Could you check a few things on this model? Use its own coordinates, in mm. A direction names the side the tool comes from. Give positions to 0.01 mm unless a question says otherwise; leave off trailing zeros. Order: outer loops, then holes, each group sorted by start corner. A loop starts at its lowest first (then second) coordinate and runs counter-clockwise, first axis right, second up. Notation, with made-up numbers: (-23.5, 31.5) -> (2.5, 31.5) arc R19 cw to (2.5, 36.5) -> close; hole circle Ø6 at (3, -26.75). An arc over 180 degrees is marked (long way). Write each question's results on one line, items separated by ' | '.
Autodesk Inventor part; units mm, degrees
ref_plane "YZ Plane" through (0, 0, 0) normal (1, 0, 0) x (0, 1, 0)
ref_plane "XZ Plane" through (0, 0, 0) normal (0, 1, 0) x (-1, 0, 0)
ref_plane "Work Plane1" through (0, 0, -3) normal (0, 0, 1) x (1, 0, 0)
sketch "Sketch1" plane through (0, 0, 0) normal (0, 0, 1) x (1, 0, 0)
  circle A0 centre (-6.35, 0) radius 3.885
  circle A1 centre (6.35, 0) radius 3.885
  arc A2 (-4.5733, 3.4549) -> (4.5733, 3.4549) centre (0, 12.3479) ccw
  line L0 (-6.35, -3.885) -> (6.35, -3.885)
  point P0 (0, 0)
  dimension "d0" = 7.77
  dimension "d1" = 6.35
  dimension "d2" = 7.77
  dimension "d3" = 6.35
  dimension "d4" = 20
  dimension "d5" = 0
  dimension "d6" = 0
extrude "Extrusion1" add sketch "Sketch1" along normal blind 1
sketch "Sketch2" plane through (0, 0, 0) normal (0, 0, -1) x (-1, 0, 0)
  arc A0 (-4.5733, 3.4549) -> (-6.35, -3.885) centre (-6.35, 0) ccw
  arc A1 (6.35, -3.885) -> (4.5733, 3.4549) centre (6.35, 0) ccw
  circle A2 centre (-6.35, 0) radius 1.9
  circle A3 centre (6.35, 0) radius 1.9
  point P0 (-4.5733, -3.4549)
  point P1 (4.5733, -3.4549)
  point P2 (0, 0)
  dimension "d10" = 3.8
  dimension "d11" = 3.8
extrude "Extrusion2" add sketch "Sketch2" along normal blind 6
sketch "Sketch3" plane through (-6.35, 0, -6) normal (0, 0, -1) x (-1, 0, 0)
  circle A0 centre (-12.7, 0) radius 1.9
  circle A1 centre (0, 0) radius 1.9
  arc A2 (-10.9233, 3.4549) -> (-1.7767, 3.4549) centre (-6.35, 12.3479) ccw
  arc A3 (-10.9233, 3.4549) -> (-12.7, -3.885) centre (-12.7, 0) ccw
  arc A4 (0, -3.885) -> (-1.7767, 3.4549) centre (0, 0) ccw
  line L0 (0, -3.885) -> (-12.7, -3.885)
  point P0 (-6.35, 0)
extrude "Extrusion3" add sketch "Sketch3" along normal blind 1 contours A0 | A1 | A2 A4 L0 A3
sketch "Sketch4" plane through (0, 0, 1) normal (0, 0, 1) x (1, 0, 0)
  arc A0 (-4.5733, 3.4549) -> (-6.35, -3.885) centre (-6.35, 0) ccw
  arc A1 (6.35, -3.885) -> (4.5733, 3.4549) centre (6.35, 0) ccw
  circle A2 centre (-6.35, 0) radius 1.3
  circle A3 centre (6.35, 0) radius 1.3
  point P0 (-4.5733, -3.4549)
  point P1 (4.5733, -3.4549)
  point P2 (0, 0)
  dimension "d16" = 2.6
  dimension "d17" = 2.6
extrude "Extrusion4" add sketch "Sketch4" along normal blind 1
sketch "Sketch5" plane through (-6.35, 0, -7) normal (0, 0, -1) x (-1, 0, 0)
  arc A0 (-10.9233, 3.4549) -> (-12.7, -3.885) centre (-12.7, 0) ccw
  arc A1 (0, -3.885) -> (-1.7767, 3.4549) centre (0, 0) ccw
  circle A2 centre (-12.7, 0) radius 1.3
  circle A3 centre (0, 0) radius 1.3
  point P0 (-10.9233, -3.4549)
  point P1 (-1.7767, -3.4549)
  point P2 (-6.35, 0)
  dimension "d20" = 2.6
  dimension "d21" = 2.6
extrude "Extrusion5" add sketch "Sketch5" along normal blind 1
chamfer "Chamfer1" distance 0.1 angle 45 2 edges at (7.65, 0, -8) (-5.05, 0, -8)
chamfer "Chamfer2" distance 0.1 angle 45 2 edges at (5.05, 0, 2) (-7.65, 0, 2)
ref_plane "Work Plane1" through (0, 0, -3) normal (0, 0, 1) x (1, 0, 0)
sketch "Skizze6" plane through (-6.35, -3.885, 0) normal (0, -1, 0) x (1, 0, 0)
  line L0 (0, 0) -> (12.7, 0)
  line L1 (12.7, 0) -> (12.7, 5)
  line L2 (12.7, 5) -> (0, 5)
  line L3 (0, 5) -> (0, 0)
  line L4 (0, -6) -> (0, -7)
  line L5 (0, -6) -> (12.7, -6)
  line L6 (12.7, -6) -> (12.7, -11)
  line L7 (12.7, -11) -> (0, -11)
  line L8 (0, -11) -> (0, -6)
  point P0 (6.35, 0)
  dimension "d31" = 5
  dimension "d32" = 12.7
  dimension "d33" = 12.7
  dimension "d34" = 5
extrude "Extrusion6" add sketch "Skizze6" along normal blind 1
sketch "Skizze7" plane through (-6.35, -4.885, 0) normal (0, -1, 0) x (1, 0, 0)
  line L0 (6.35, 0) -> (6.35, 2.5)
  line L1 (6.35, 2.5) -> (3.175, 2.5)
  line L2 (6.35, 2.5) -> (9.525, 2.5)
  line L3 (10.9233, -6) -> (1.7767, -6)
  line L4 (6.35, -6) -> (6.35, -8.5)
  line L5 (6.35, -8.5) -> (3.175, -8.5)
  line L6 (6.35, -8.5) -> (9.525, -8.5)
  dimension "d37" = 2.5
  dimension "d38" = 3.175
  dimension "d39" = 3.175
  dimension "d40" = 2.5
  dimension "d41" = 3.175
  dimension "d42" = 3.175
hole "Bohrung1" at (3.175, -4.885, -8.5) at (-3.175, -4.885, -8.5) at (3.175, -4.885, 2.5) at (-3.175, -4.885, 2.5) direction (0, 1, 0) diameter 1 end through all
equation "\"d2\" = d0"
equation "\"d11\" = d10"
equation "\"d17\" = d16"
equation "\"d20\" = d16"
equation "\"d21\" = d16"
properties part number "ConnectingLinks"
Q1. Suppose I cut it at A-A on z = 2.5. Please give me the cut outline in (x, y) (3 decimals), and give its area (3 significant figures).
Here are the results:
outline: (-6.35, -4.885) -> (-3.675, -4.885) -> (-3.675, -3.885) -> (-6.35, -3.885) -> close; (-2.675, -4.885) -> (2.675, -4.885) -> (2.675, -3.885) -> (-2.675, -3.885) -> close; (3.675, -4.885) -> (6.35, -4.885) -> (6.35, -3.885) -> (3.675, -3.885) -> close | area: 10.7 mm²
Q2. Suppose I cut it at C-C on x = -1.25. Please give me the cut outline in (y, z) (3 decimals), and give its area (3 significant figures).
Here are the results:
outline: (-4.885, -11) -> (-3.885, -11) -> (-3.885, -7) -> (2.426, -7) -> (2.426, -6) -> (-4.885, -6) -> close; (-4.885, 0) -> (2.426, 0) -> (2.426, 1) -> (-3.885, 1) -> (-3.885, 5) -> (-4.885, 5) -> close | area: 22.6 mm²
Q3. I need wall thicknesses on line 1 along X through (y, z) = (-4.4, -8.5) (3 decimals); line 2 along Z through (x, y) = (7.75, -3); line 3 along Y through (x, z) = (2.75, 4.5) (3 decimals). Which ranges of each line are inside material? Lowest first, please.
Here are the results:
line 1: x = -6.35 to -3.675, -2.675 to 2.675, 3.675 to 6.35 | line 2: z = -7 to -6, 0 to 1 | line 3: y = -4.885 to -3.885
Q4. Suppose I cut it at B-B on z = -1.25. Please give me the cut outline in (x, y), and give its area (3 significant figures).
Here are the results:
outline: circle Ø3.8 at (-6.35, 0); circle Ø3.8 at (6.35, 0) | area: 22.7 mm²
Q5. Thinking about a two-plate mould opening in Y: for faces 1 (the cylindrical face through (-5.05, -0.06, -7.44)), 2 (the cylindrical face through (10.1, 1.01, 0.49)), 3 (the cylindrical face through (-2.98, -4.38, -8.96)), which applies, +Y half, -Y half, draft (parallel to the pull), parting line (faces both ways), or undercut?
Here are the results:
face 1: undercut | face 2: parting line | face 3: draft
Q6. Suppose I cut it at D-D on z = 0.5. Please give me the cut outline in (x, y) (3 decimals).
Here are the results:
outline: (-6.35, -4.885) -> (6.35, -4.885) -> (6.35, -3.885) arc R3.885 ccw (long way) to (4.573, 3.455) arc R10 cw to (-4.573, 3.455) arc R3.885 ccw (long way) to (-6.35, -3.885) -> close
Q7. I'm going to push flat-ended pins straight in: pin 1 Ø0.5 at (y, z) = (-4.5, 3.5) entering from +X; pin 2 Ø1.5 at (x, y) = (2, 1) entering from -Z; pin 3 Ø0.7 at (x, y) = (-6.5, -0.5) entering from -Z; pin 4 Ø4.5 at (x, y) = (3, -2.5) entering from -Z. Where does each tip first touch, or does it pass through?
Here are the results:
pin 1: stops at x = 6.35 | pin 2: stops at z = -7 | pin 3: stops at z = -8 | pin 4: stops at z = -11
Q8. For faces 4 (the cylindrical face through (-4.45, -0.08, -2.96)), 5 (the flat face through (-6, 0, -8)), 6 (the cylindrical face through (-0.07, 2.35, -6.49)), 7 (the flat face through (0.1, -4.4, 5)), 8 (the flat face through (-6, 0, 2)), which set-ups out of +Z, -Z, +X, -X, +Y, -Y let a thin tool reach every point of the face, with its end or its side?
Here are the results:
face 4: none | face 5: -Z, +X, -X, +Y | face 6: +Z, -Z, +Y | face 7: +Z, +X, -X, +Y, -Y | face 8: +Z, +X, -X, +Y
